```python
from build123d import *

# Parameters (mm, degrees)
SKETCH_1_R          = 1.6
EXTRUDE_1_DEPTH     = 2
SKETCH_2_W          = 16
SKETCH_2_H          = 13.5
SKETCH_2_W_2        = 3
SKETCH_2_H_2        = 1
CUT_EXTRUDE_2_DEPTH = 2
SKETCH_3_W          = 20
SKETCH_3_H          = 2.5
EXTRUDE_2_DEPTH     = 20
CUT_EXTRUDE_3_DEPTH = 20
SKETCH_6_W          = 20
SKETCH_6_H          = 2.5
CUT_EXTRUDE_4_DEPTH = 20


with BuildPart() as part:
    # 草图1 → 凸台-拉伸1 (new body)
    with BuildSketch(Plane.XY):
        with BuildLine():
            Line((3, 0), (68, 0))
            ThreePointArc((68, 0), (70.121320344, -0.878679656), (71, -3))
            Line((71, -3), (71, -23.6))
            ThreePointArc((71, -23.6), (70.121320344, -25.721320344), (68, -26.6))
            Line((68, -26.6), (3, -26.6))
            ThreePointArc((3, -26.6), (0.878679656, -25.721320344), (0, -23.6))
            Line((0, -23.6), (0, -3))
            ThreePointArc((0, -3), (0.878679656, -0.878679656), (3, 0))
        make_face()
        with Locations((3, -3)):
            Circle(SKETCH_1_R, mode=Mode.SUBTRACT)
        with Locations((68, -3)):
            Circle(SKETCH_1_R, mode=Mode.SUBTRACT)
        with Locations((68, -23.6)):
            Circle(SKETCH_1_R, mode=Mode.SUBTRACT)
        with Locations((3, -23.6)):
            Circle(SKETCH_1_R, mode=Mode.SUBTRACT)
    extrude(amount=EXTRUDE_1_DEPTH)

    # 草图2 → 切除-拉伸2 (cut)
    with BuildSketch(Plane(origin=(0, 0, 0), x_dir=(-1, 0, 0), z_dir=(0, 0, -1))):
        with Locations((-51, -10.25)):
            Rectangle(SKETCH_2_W, SKETCH_2_H)
        with BuildLine():
            Line((-19.7, -17), (-13.1, -17))
            ThreePointArc((-13.1, -17), (-12.180761184, -16.619238816), (-11.8, -15.7))
            Line((-11.8, -15.7), (-11.8, -14.9))
            ThreePointArc((-11.8, -14.9), (-12.180761184, -13.980761184), (-13.1, -13.6))
            Line((-13.1, -13.6), (-19.7, -13.6))
            ThreePointArc((-19.7, -13.6), (-20.619238816, -13.980761184), (-21, -14.9))
            Line((-21, -14.9), (-21, -15.7))
            ThreePointArc((-21, -15.7), (-20.619238816, -16.619238816), (-19.7, -17))
        make_face()
        with Locations((-39.084, -16.5)):
            Rectangle(SKETCH_2_W_2, SKETCH_2_H_2)
        with Locations((-34.343, -16.5)):
            Rectangle(SKETCH_2_W_2, SKETCH_2_H_2)
        with Locations((-29.601, -16.5)):
            Rectangle(SKETCH_2_W_2, SKETCH_2_H_2)
        with Locations((-24.86, -16.5)):
            Rectangle(SKETCH_2_W_2, SKETCH_2_H_2)
    extrude(amount=-CUT_EXTRUDE_2_DEPTH, mode=Mode.SUBTRACT)

    # 草图3 → 凸台-拉伸2 (add)
    with BuildSketch(Plane.XY.offset(2)):
        with Locations((22, -3)):
            Rectangle(SKETCH_3_W, SKETCH_3_H)
    extrude(amount=EXTRUDE_2_DEPTH)

    # 草图5 → 切除-拉伸3 (cut)
    with BuildSketch(Plane.XY.offset(2)):
        with BuildLine():
            Line((14.347228721, -10.5), (16, -4.25))
            Line((16, -4.25), (13, -4.25))
            ThreePointArc((13, -4.25), (12.292893219, -4.542893219), (12, -5.25))
            Line((12, -5.25), (12, -9.5))
            ThreePointArc((12, -9.5), (12.292893219, -10.207106781), (13, -10.5))
            Line((13, -10.5), (14.347228721, -10.5))
        make_face()
        Polygon((22.325, -4.25), (17, -4.25), (15.347228721, -10.5), (20.672228721, -10.5), align=None)
        Polygon((28.652771279, -4.25), (23.325, -4.25), (21.672228721, -10.5), (27, -10.5), align=None)
        with BuildLine():
            Line((31, -4.25), (29.652771279, -4.25))
            Line((29.652771279, -4.25), (28, -10.5))
            Line((28, -10.5), (31, -10.5))
            ThreePointArc((31, -10.5), (31.707106781, -10.207106781), (32, -9.5))
            Line((32, -9.5), (32, -5.25))
            ThreePointArc((32, -5.25), (31.707106781, -4.542893219), (31, -4.25))
        make_face()
    extrude(amount=-CUT_EXTRUDE_3_DEPTH, mode=Mode.SUBTRACT)

    # 草图6 → 切除-拉伸4 (cut)
    with BuildSketch(Plane.XY.offset(22)):
        with Locations((22, -3)):
            Rectangle(SKETCH_6_W, SKETCH_6_H)
    extrude(amount=-CUT_EXTRUDE_4_DEPTH, mode=Mode.SUBTRACT)


solid = part.part
```
Model file for the job. Use its own axes, mm. A direction names the side the tool comes from. Coordinates: 2 decimals unless noted, no trailing zeros. Loops run counter-clockwise (first coordinate to the right, second up) from the corner with the lowest first, then second, coordinate; pieces in that order, holes last. Notation, with made-up numbers: (19, 31.5) -> (50, 31.5) arc R17 cw to (50, 51.5) -> close; hole circle Ø4 at (-8, -25.5). An arc over 180 degrees is marked (long way). Answer as a JSON object with one key per item and string values.
Q1. Probe probe 1 along Y at (x, z) = (19, 1.15); probe 2 along Y at (x, z) = (68, 1.3); probe 3 along X at (y, z) = (-15, 1.35). List the from-to ranges inside material, lowest first.
Report:
{"probe 1": "y = -26.6 to -17, -13.6 to -10.5, -4.25 to 0", "probe 2": "y = -26.6 to -25.2, -22 to -4.6, -1.4 to 0", "probe 3": "x = 0 to 11.8, 21 to 43, 59 to 71"}
Q2. Cut at B-B (x = 48.5). List the corners of the cut face in (y, z).
Report:
{"outline": "(-26.6, 0) -> (-17, 0) -> (-17, 2) -> (-26.6, 2) -> close; (-3.5, 0) -> (0, 0) -> (0, 2) -> (-3.5, 2) -> close"}
Q3. Cut at A-A (y = -12.5). List the corners of the cut face in (x, z).
Report:
{"outline": "(0, 0) -> (43, 0) -> (43, 2) -> (0, 2) -> close; (59, 0) -> (71, 0) -> (71, 2) -> (59, 2) -> close"}
Q4. Pull direction X, two halves, no side cores. Call faces 1 (the flat face through (24, -10.5, 1)), 2 (the cylindrical face through (70.14, -25.7, 0.99)), 3 (the flat face through (36, -13, 2)): released by +X, released by -X, zero draft, split by the parting line, or undercut.
Report:
{"face 1": "undercut", "face 2": "released by +X", "face 3": "zero draft"}
Q5. 3-axis set-ups, long thin cutter, end or side, ignore diameter. For faces 4 (the flat face through (35, 0, 1)), 5 (the flat face through (59, -10, 1)): which of +Z, -Z, +X, -X, +Y, -Y reach the whole face in a straight line?
Report:
{"face 4": "+Z, -Z, +X, -X, +Y", "face 5": "+Z, -Z"}
